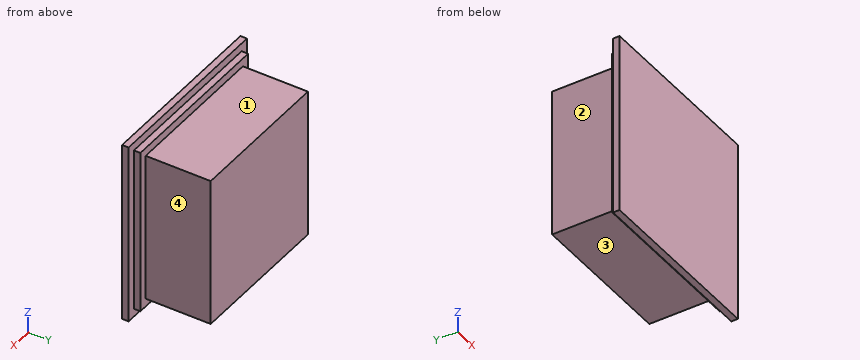
```python
from build123d import *

# Parameters (mm, degrees)
SKETCH1_W           = 28
SKETCH1_H           = 28
BOSS_EXTRUDE1_DEPTH = 1
SKETCH2_W           = 25.5
SKETCH2_H           = 25.5
BOSS_EXTRUDE2_DEPTH = 1
SKETCH3_W           = 23
SKETCH3_H           = 23
BOSS_EXTRUDE3_DEPTH = 10


with BuildPart() as part:
    # Sketch1 → Boss-Extrude1 (new body)
    with BuildSketch(Plane(origin=(0, 0, 0), x_dir=(1, 0, 0), z_dir=(0, 1, 0))):
        Rectangle(SKETCH1_W, SKETCH1_H)
    extrude(amount=BOSS_EXTRUDE1_DEPTH)

    # Sketch2 → Boss-Extrude2 (add)
    with BuildSketch(Plane(origin=(0, 1, 0), x_dir=(1, 0, 0), z_dir=(0, 1, 0))):
        Rectangle(SKETCH2_W, SKETCH2_H)
    extrude(amount=BOSS_EXTRUDE2_DEPTH)

    # Sketch3 → Boss-Extrude3 (add)
    with BuildSketch(Plane(origin=(0, 2, 0), x_dir=(1, 0, 0), z_dir=(0, 1, 0))):
        Rectangle(SKETCH3_W, SKETCH3_H)
    extrude(amount=BOSS_EXTRUDE3_DEPTH)


solid = part.part
```
Source: CAD feature listing. Evaluate the final solid. Frame: model axes, mm. Face numbers are marked on the shaded views. A direction names the side the tool comes from. Give positions to 0.01 mm unless a question says otherwise; leave off trailing zeros. Order: outer loops, then holes, each group sorted by start corner. A loop starts at its lowest first (then second) coordinate and runs counter-clockwise, first axis right, second up.
(1) Section query B-B (x = 9.25). Return the cut outline in (y, z), plus the area to 4 significant figures.
(2) Section query C-C (y = 8). Return the cut outline in (x, z).
(3) Contact query for flat-ended pins moving along their axis: P1, Ø0.5, axis at x = -2, y = 1.5, coming from the +Z side; P2, Ø5, axis at x = 7.5, y = 9.5, coming from the +Z side; P3, Ø1.5, axis at y = 2, z = -11, coming from the -X side. Output: stop coordinate, or through.
(4) Access query for the marked faces 1, 2, 3 and 4. Directions: +Z, -Z, +X, -X, +Y, -Y. A direction counts if a zero-diameter tool reaches every point of the face in a straight line with its end or side. Return the directions, or none.
(5) Material intervals for line 1 along X through (y, z) = (4.25, 2); line 2 along Y through (x, z) = (9.5, 12.5), sorted ascending.
(6) Section query A-A (z = 0.5). Return the cut outline in (x, y).
Outcome:
1. outline: (0, -14) - (1, -14) - (1, -12.75) - (2, -12.75) - (2, -11.5) - (12, -11.5) - (12, 11.5) - (2, 11.5) - (2, 12.75) - (1, 12.75) - (1, 14) - (0, 14) - close
1. area: 283.5 mm2
2. outline: (-11.5, -11.5) - (11.5, -11.5) - (11.5, 11.5) - (-11.5, 11.5) - close
3. P1: stops at z = 12.75
3. P2: stops at z = 11.5
3. P3: stops at x = -12.75
4. face 1: +Z, +X, -X, +Y
4. face 2: +Z, -Z, -X, +Y
4. face 3: -Z, +X, -X, +Y
4. face 4: +Z, -Z, +X, +Y
5. line 1: x = -11.5 to 11.5
5. line 2: y = 0 to 2
6. outline: (-14, 0) - (14, 0) - (14, 1) - (12.75, 1) - (12.75, 2) - (11.5, 2) - (11.5, 12) - (-11.5, 12) - (-11.5, 2) - (-12.75, 2) - (-12.75, 1) - (-14, 1) - close
